The model under review builds one solid part; all positions refer to its coordinate system, in mm. A direction names the side the tool comes from. Coordinates: 2 decimals unless noted, no trailing zeros. Loops run counter-clockwise (first coordinate to the right, second up) from the corner with the lowest first, then second, coordinate; pieces in that order, holes last. Notation, with made-up numbers: (9, -6) - (66, -6) arc R17 cw to (66, 7) - close; hole circle Ø5 at (12.25, 11.5). An arc over 180 degrees is marked (long way). Answer in a Markdown table with one row per item. Add a question column.
(1) Machinability: for faces 1 (the flat face through (0, -28, 30.711)), 2 (the cylindrical face through (-3.902, 112.7, 29.717)), which of the approach directions +Z, -Z, +X, -X, +Y, -Y give a long, thin tool a straight path to every point of the face, cutting with its end or side? Answer none if there is none.
(2) For P1, Ø12, axis at x = -4, y = 144.5, coming from the +Z side; P2, Ø5, axis at x = -15.5, y = 31, coming from the -Z side; P3, Ø2, axis at x = 19.5, y = 110, coming from the -Z side, all flat-tipped, find the tip position at first contact; note any pin that passes through.
(3) We need section C-C on z = -20. Write out the cut boundary in (x, y), plus the area to 3 significant figures.
(4) For line 1 along Z through (x, y) = (-1.5, 198); line 2 along Z through (x, y) = (-21, -32); line 3 along Y through (x, z) = (-26, -22), list the stretches that pass through material, from the lowest coordinate up.
(5) Mouldability with a two-part tool opening along Z and no side actions: class faces 3 (the cylindrical face through (0.43, -8.125, -9.364)), 4 (the flat face through (30.709, -5, 2)), 5 (the cylindrical face through (0.36, -59.97, 29.18)) as +Z half, -Z half, draft (parallel to the pull), parting line (faces both ways), or undercut.
(6) We need section B-B on x = 0. Write out the cut boundary in (y, z) (1 decimal).
(7) We need section A-A on z = 0. Write out the cut boundary in (x, y), plus the area to 3 significant figures.
(8) We need section D-D on x = 13. Write out the cut boundary in (y, z) (1 decimal).
from build123d import *

# Parameters (mm, degrees)
F0_R     = 29.972
F1_DEPTH = 228.6
F2_W     = 61.4172
F2_H     = 61.4225
F3_DEPTH = 61.4172
F5_D     = 48.895
F6_R     = 5.08


with BuildPart() as f1:
    # F0 (on Front) → F1 (new body)
    with BuildSketch(Plane.XZ):
        Circle(F0_R)
    extrude(amount=-F1_DEPTH)

    # F2 (on Front) → F3 (join)
    with BuildSketch(Plane.XZ):
        Rectangle(F2_W, F2_H)
    extrude(amount=F3_DEPTH)

    # F5 (through all)
    with Locations(Plane(origin=(-30.7086, 0, 0), x_dir=(0, -1, 0), z_dir=(-1, 0, 0))):
        with Locations((30.7086, 0)):
            Hole(F5_D / 2)

    # F6
    f6_edges = [f1.edges().sort_by_distance(p)[0] for p in [
        (-30.7086, -30.7086, 30.71125),
        (0, -61.4172, 30.71125),
        (-30.7086, -61.4172, 0),
        (30.7086, -30.7086, 30.71125),
        (30.7086, -61.4172, 0),
        (30.7086, -30.7086, -30.71125),
        (0, -61.4172, -30.71125),
        (-30.7086, -30.7086, -30.71125),
    ]]
    fillet(f6_edges, radius=F6_R)


solid = f1.part
Outcome:
| question | item | result |
|---|---|---|
| 1 | face 1 | +Z, +X, -X, +Y, -Y |
| 1 | face 2 | +Y |
| 2 | P1 | z = 29.97 |
| 2 | P2 | z = -27.01 |
| 2 | P3 | z = -23.58 |
| 3 | outline | (-30.71, -56.34) arc R5.08 ccw to (-25.63, -61.42) - (25.63, -61.42) arc R5.08 ccw to (30.71, -56.34) - (30.71, -44.77) - (-30.71, -44.77) - close; (-30.71, -16.65) - (30.71, -16.65) - (30.71, 0) - (22.32, 0) - (22.32, 228.6) - (-22.32, 228.6) - (-22.32, 0) - (-30.71, 0) - close |
| 3 | area | 12,200 mm² |
| 4 | line 1 | -29.93 to 29.93 |
| 4 | line 2 | -30.71 to -24.41, 24.41 to 30.71 |
| 4 | line 3 | -61.4 to -41.37, -20.05 to 0 |
| 5 | face 3 | undercut |
| 5 | face 4 | draft |
| 5 | face 5 | +Z half |
| 6 | outline | (-61.4, -25.6) arc R5.1 ccw to (-56.3, -30.7) - (0, -30.7) - (0, -30) - (228.6, -30) - (228.6, 30) - (0, 30) - (0, 30.7) - (-56.3, 30.7) arc R5.1 ccw to (-61.4, 25.6) - close; hole circle Ø48.9 at (-30.7, 0) |
| 7 | outline | (-30.71, -56.34) arc R5.08 ccw to (-25.63, -61.42) - (25.63, -61.42) arc R5.08 ccw to (30.71, -56.34) - (30.71, -55.16) - (-30.71, -55.16) - close; (-30.71, -6.26) - (30.71, -6.26) - (30.71, 0) - (29.97, 0) - (29.97, 228.6) - (-29.97, 228.6) - (-29.97, 0) - (-30.71, 0) - close |
| 7 | area | 14,500 mm² |
| 8 | outline | (-61.4, -25.6) arc R5.1 ccw to (-56.3, -30.7) - (0, -30.7) - (0, -27) - (228.6, -27) - (228.6, 27) - (0, 27) - (0, 30.7) - (-56.3, 30.7) arc R5.1 ccw to (-61.4, 25.6) - close; hole circle Ø48.9 at (-30.7, 0) |
